Verification items for the finished model (mm, model axes). Face numbers are marked on the shaded views. A direction names the side the tool comes from. Give positions to 0.01 mm unless a question says otherwise; leave off trailing zeros. Order: outer loops, then holes, each group sorted by start corner. A loop starts at its lowest first (then second) coordinate and runs counter-clockwise, first axis right, second up. Notation, with made-up numbers: (79, 13) -> (107, 13) arc R18 ccw to (107, 17) -> close; hole circle Ø6 at (30, 59). An arc over 180 degrees is marked (long way). Write each question's results on one line, items separated by ' | '. Start each with the question number.
1. Cross-section at B-B, the plane x = 5. Enter the section's corners in (y, z).
2. Cross-section at D-D, the plane x = 4. Enter the section's corners in (y, z).
3. Mould release check, pull along Y, two halves, no side actions. Record for the marked faces 1, 2, 3 and 4: +Y half, -Y half, draft (parallel to the pull), parting line (faces both ways), or undercut.
4. Set-up check for the marked faces 5 and 6: record each of +Z, -Z, +X, -X, +Y, -Y from which the full face is reachable in a straight line by a thin tool's end or side.
5. Cross-section at A-A, the plane y = -6. Enter the section's corners in (x, z), then the cut area to 3 significant figures.
6. Material ranges on L1, parallel to Y at x = 5, z = 1.9; L2, parallel to Y at x = 4, z = 6.25; L3, parallel to Z at x = 4, y = -7.25, recorded low to high. Write a range as from..to.
7. Cross-section at C-C, the plane z = 0.75. Enter the section's corners in (x, y).
from build123d import *

# Parameters (mm, degrees)
F0_W     = 10
F0_H     = 10
F1_DEPTH = 8
F2_W     = 4.5
F2_H     = 5.2
F3_DEPTH = 2
F4_R     = 0.5
F5_DEPTH = 25


with BuildPart() as f1:
    # F0 (on Top) → F1 (new body)
    with BuildSketch(Plane.XY):
        with Locations((5, -5)):
            Rectangle(F0_W, F0_H)
    extrude(amount=F1_DEPTH)

    # F2 (on face) → F3 (cut)
    with BuildSketch(Plane.XY.offset(8)):
        with Locations((5, -5)):
            Rectangle(F2_W, F2_H)
    extrude(amount=-F3_DEPTH, mode=Mode.SUBTRACT)

    # F4 (on face) → F5 (cut)
    with BuildSketch(Plane.XY.offset(6)):
        with Locations((5, -4)):
            Circle(F4_R)
        with Locations((5, -6)):
            Circle(F4_R)
    extrude(amount=-F5_DEPTH, mode=Mode.SUBTRACT)


solid = f1.part
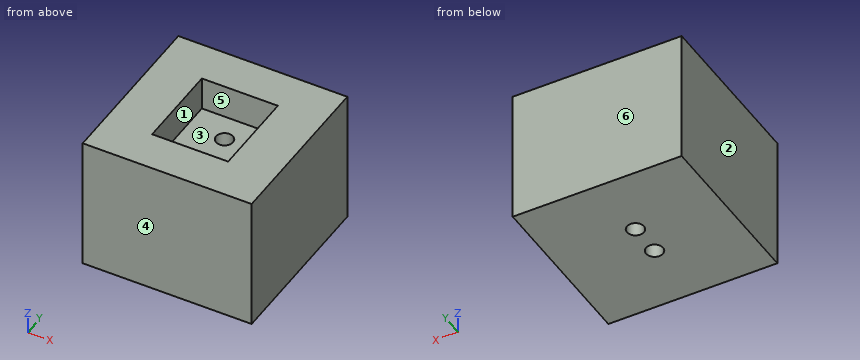
Results below:
1) outline: (-10, 0) -> (-6.5, 0) -> (-6.5, 6) -> (-7.6, 6) -> (-7.6, 8) -> (-10, 8) -> close; (-5.5, 0) -> (-4.5, 0) -> (-4.5, 6) -> (-5.5, 6) -> close; (-3.5, 0) -> (0, 0) -> (0, 8) -> (-2.4, 8) -> (-2.4, 6) -> (-3.5, 6) -> close
2) outline: (-10, 0) -> (0, 0) -> (0, 8) -> (-2.4, 8) -> (-2.4, 6) -> (-7.6, 6) -> (-7.6, 8) -> (-10, 8) -> close
3) face 1: undercut | face 2: draft | face 3: undercut | face 4: -Y half
4) face 5: +Z | face 6: +Z, -Z, +X, -X, +Y
5) outline: (0, 0) -> (4.5, 0) -> (4.5, 6) -> (2.75, 6) -> (2.75, 8) -> (0, 8) -> close; (5.5, 0) -> (10, 0) -> (10, 8) -> (7.25, 8) -> (7.25, 6) -> (5.5, 6) -> close | area: 65.0 mm²
6) L1: y = -10..-6.5, -5.5..-4.5, -3.5..0 | L2: y = -10..-7.6, -2.4..0 | L3: z = 0..6
7) outline: (0, -10) -> (10, -10) -> (10, 0) -> (0, 0) -> close; hole circle Ø1 at (5, -6); hole circle Ø1 at (5, -4)
